Could you check a few things on this drawing? It's one solid part, dimensions in mm from its lowest x, y, z. Give positions to 0.01 mm unless a question says otherwise; leave off trailing zeros. Order: outer loops, then holes, each group sorted by start corner. A loop starts at its lowest first (then second) coordinate and runs counter-clockwise, first axis right, second up. Notation, with made-up numbers: M -18.5,1 L 34.5,1 A22 cw 34.5,20 Z; hole C -39,7.25 d9. An arc over 180 degrees is marked long. Use one line per item in the form item = value. Start each with the question number.
1. I want a section at B-B, the plane x = 10. List the corners of the cut face in (y, z) for me, and give its area (3 significant figures).
2. I want a section at C-C, the plane z = 10. List the corners of the cut face in (x, y) for me.
3. I need wall thicknesses on L1, parallel to X at y = 2.15, z = 10; L2, parallel to Z at x = 11.5, y = 2; L3, parallel to Z at x = 36, y = 2.2. Which ranges of each line are inside material? Lowest first, please.
4. Will this pin go through, and if not, where does the flat tip stop? P1, Ø4, axis at x = 6.5, z = 5, coming from the -Y side.
5. We'd pull the mould along X, two halves only. Please class the marked faces 1, 2, 3 and 4: +X half, -X half, draft (parallel to the pull), parting line (faces both ways), or undercut.
6. I want a section at A-A, the plane y = 2.6. List the corners of the cut face in (x, z) for me, and give its area (3 significant figures).
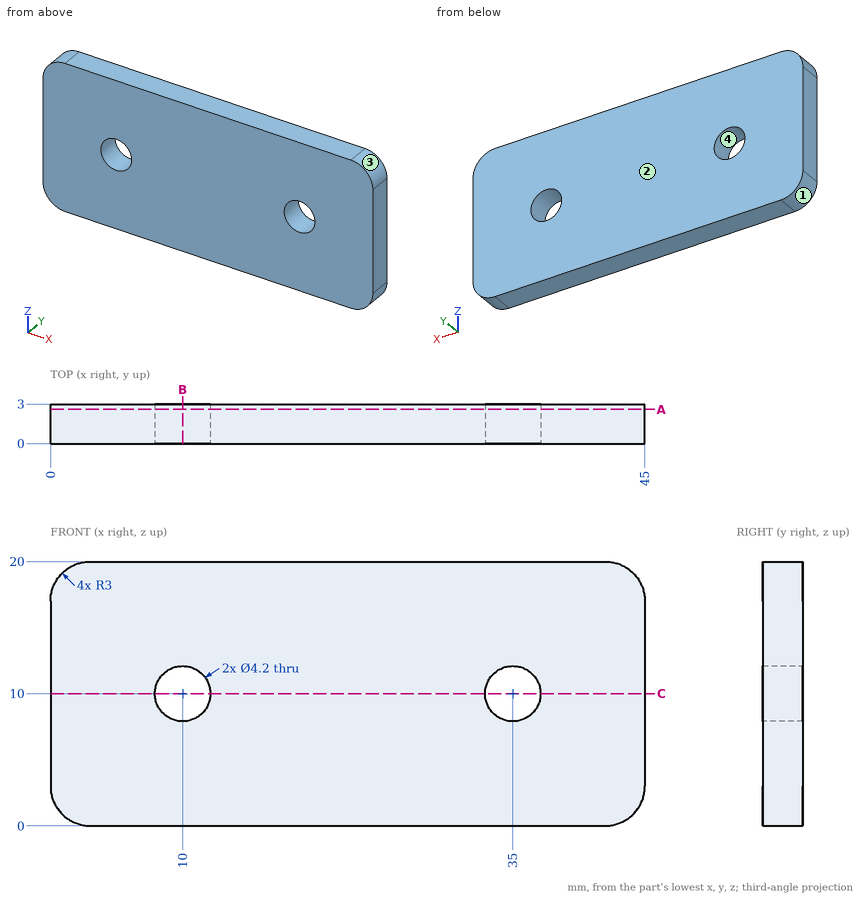
Check result:
q1.outline = M 0,0 L 3,0 L 3,7.9 L 0,7.9 Z; M 0,12.1 L 3,12.1 L 3,20 L 0,20 Z
q1.area = 47.4 mm2
q2.outline = M 0,0 L 7.9,0 L 7.9,3 L 0,3 Z; M 12.1,0 L 32.9,0 L 32.9,3 L 12.1,3 Z; M 37.1,0 L 45,0 L 45,3 L 37.1,3 Z
q3.L1 = 0 to 7.9, 12.1 to 32.9, 37.1 to 45
q3.L2 = 0 to 8.53, 11.47 to 20
q3.L3 = 0 to 8.15, 11.85 to 20
q4.P1 = 0
q5.face_1 = -X half
q5.face_2 = draft
q5.face_3 = +X half
q5.face_4 = undercut
q6.outline = M 0,3 A3 ccw 3,0 L 42,0 A3 ccw 45,3 L 45,17 A3 ccw 42,20 L 3,20 A3 ccw 0,17 Z; hole C 10,10 d4.2; hole C 35,10 d4.2
q6.area = 865 mm2
